For this review, take the finished solid that the model builds, in its own axes (mm). Coordinates: 2 decimals unless noted, no trailing zeros. Write each loop counter-clockwise with the first axis right and the second up, starting at its lowest first coordinate (ties: lowest second). Pieces come first, ordered by that corner, then holes. Notation, with made-up numbers: M 19.25,16 L 41.25,16 A14 ccw 41.25,43 Z; hole C 40.25,47 d1. An arc over 180 degrees is marked long. One line per question, with ' | ' between items.
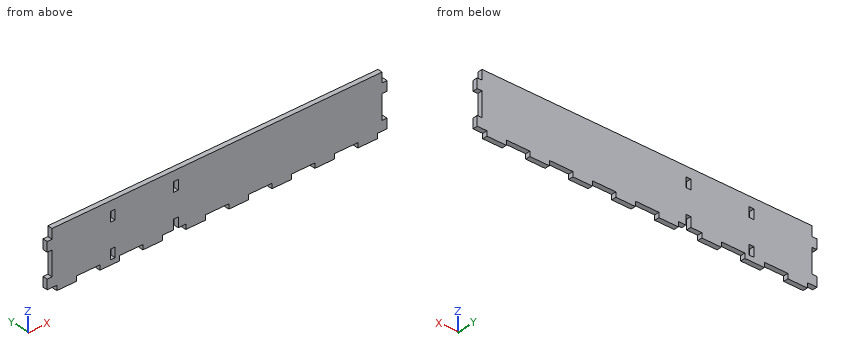
from build123d import *

# Parameters (mm, degrees)
F0_W     = 444.5
F0_H     = 76.2
F1_DEPTH = 6.35
F2_W     = 6.35
F2_H     = 6.35
F2_H_2   = 12.7
F2_H_3   = 31.75
F3_DEPTH = 6.35
F4_W     = 30.842857
F4_H     = 6.35
F4_W_2   = 30.842858
F4_W_3   = 6.35
F5_DEPTH = 6.351
F6_W     = 6.35
F6_H     = 12.7
F7_DEPTH = 6.351


with BuildPart() as f1:
    # F0 (on Front) → F1 (new body)
    with BuildSketch(Plane.XZ):
        with Locations((222.25, 38.1)):
            Rectangle(F0_W, F0_H)
    extrude(amount=F1_DEPTH)

    # F2 (on face) → F3 (cut, through all)
    with BuildSketch(Plane.XZ.offset(6.35)):
        with Locations((3.175, 3.175)):
            Rectangle(F2_W, F2_H)
        with Locations((3.175, 69.85)):
            Rectangle(F2_W, F2_H_2)
        with Locations((3.175, 34.925)):
            Rectangle(F2_W, F2_H_3)
        with Locations((441.325, 3.175)):
            Rectangle(F2_W, F2_H)
        with Locations((441.325, 34.925)):
            Rectangle(F2_W, F2_H_3)
        with Locations((441.325, 69.85)):
            Rectangle(F2_W, F2_H_2)
    extrude(amount=-F3_DEPTH, mode=Mode.SUBTRACT)

    # F4 (on face) → F5 (cut, through all)
    with BuildSketch(Plane.XZ.offset(6.35)):
        with Locations((53.521428, 3.175)):
            Rectangle(F4_W, F4_H)
        with Locations((109.764285, 3.175)):
            Rectangle(F4_W, F4_H)
        with Locations((166.007142, 3.175)):
            Rectangle(F4_W, F4_H)
        with Locations((222.25, 3.175)):
            Rectangle(F4_W_2, F4_H)
        with Locations((278.492858, 3.175)):
            Rectangle(F4_W, F4_H)
        with Locations((334.735714, 3.175)):
            Rectangle(F4_W, F4_H)
        with Locations((390.978571, 3.175)):
            Rectangle(F4_W, F4_H)
        with Locations((9.525, 3.175)):
            Rectangle(F4_W_3, F4_H)
        with Locations((434.975, 3.175)):
            Rectangle(F4_W_3, F4_H)
    extrude(amount=-F5_DEPTH, mode=Mode.SUBTRACT)

    # F6 (on face) → F7 (cut, through all)
    with BuildSketch(Plane.XZ.offset(6.35)):
        with Locations((85.725, 12.7)):
            Rectangle(F6_W, F6_H)
        with Locations((85.725, 57.15)):
            Rectangle(F6_W, F6_H)
        with Locations((168.275, 12.7)):
            Rectangle(F6_W, F6_H)
        with Locations((168.275, 57.15)):
            Rectangle(F6_W, F6_H)
    extrude(amount=-F7_DEPTH, mode=Mode.SUBTRACT)


solid = f1.part
1) We need section C-C on x = 270.5. State the section outline as (y, z) points.
Responses:
outline: M -6.35,6.35 L 0,6.35 L 0,76.2 L -6.35,76.2 Z
2) Insertion check: pin 1 Ø1.9 at (x, y) = (441, -5) entering from -Z; pin 2 Ø3 at (y, z) = (-3.5, 4.5) entering from +X. Each pin has a flat end and moves straight along its axis. Give the tip position at first contact, or say it passes through.
Responses:
pin 1: z = 6.35 | pin 2: x = 431.8
3) We need section B-B on y = -1.25. State how many separate pieces and enclosed holes the cut face has, then the cut area to 3 significant figures.
Responses:
separate pieces: 1 | enclosed holes: 3 | area: 31,500 mm^2
4) To check wall thickness, follow line 1 along X through (y, z) = (-4.75, 57.5); line 2 along Z through (x, y) = (403.5, -4.5); line 3 along X through (y, z) = (-3.25, 43). State the ranges of each line that lie inside material, in increasing order. Write a range as [from, to].
Responses:
line 1: [0, 82.55], [88.9, 165.1], [171.45, 444.5] | line 2: [6.35, 76.2] | line 3: [6.35, 438.15]
5) We need section D-D on z = 46. State the section outline as (x, y) points.
Responses:
outline: M 6.35,-6.35 L 438.15,-6.35 L 438.15,0 L 6.35,0 Z
6) We need section A-A on z = 10. State the section outline as (x, y) points.
Responses:
outline: M 0,-6.35 L 82.55,-6.35 L 82.55,0 L 0,0 Z; M 88.9,-6.35 L 165.1,-6.35 L 165.1,0 L 88.9,0 Z; M 171.45,-6.35 L 444.5,-6.35 L 444.5,0 L 171.45,0 Z
